from build123d import *

# Parameters (mm, degrees)
SKETCH1_R             = 8
BOSS_EXTRUDE1_DEPTH   = 7
SKETCH2_R             = 6
BOSS_EXTRUDE2_DEPTH   = 7
SKETCH3_R             = 8
BOSS_EXTRUDE3_DEPTH   = 2
CHAMFER1_SIZE         = 0.2
SKETCH4_R             = 2.5
CUT_EXTRUDE1_DEPTH    = 20
BODY_MOVE_COPY1_ANGLE = 180
CUT_EXTRUDE2_DEPTH    = 3


with BuildPart() as part:
    # Sketch1 → Boss-Extrude1 (new body)
    with BuildSketch(Plane(origin=(0, 0, 0), x_dir=(1, 0, 0), z_dir=(0, 1, 0))):
        with Locations(Location((0, 0, 0), (0, 0, 270))):
            Circle(SKETCH1_R)
    extrude(amount=BOSS_EXTRUDE1_DEPTH)

    # Sketch2 → Boss-Extrude2 (add)
    with BuildSketch(Plane(origin=(0, 7, 0), x_dir=(1, 0, 0), z_dir=(0, 1, 0))):
        with Locations(Location((0, 0, 0), (0, 0, 270))):
            Circle(SKETCH2_R)
    extrude(amount=BOSS_EXTRUDE2_DEPTH)

    # Sketch3 → Boss-Extrude3 (add)
    with BuildSketch(Plane(origin=(0, 14, 0), x_dir=(1, 0, 0), z_dir=(0, 1, 0))):
        with Locations(Location((0, 0, 0), (0, 0, 270))):
            Circle(SKETCH3_R)
    extrude(amount=BOSS_EXTRUDE3_DEPTH)

    # Chamfer1
    chamfer1_edges = [part.edges().sort_by_distance(p)[0] for p in [
        (0, 0, -8),
        (0, 7, -8),
        (0, 14, -8),
        (0, 16, -8),
    ]]
    chamfer(chamfer1_edges, length=CHAMFER1_SIZE)

    # Sketch4 → Cut-Extrude1 (cut)
    with BuildSketch(Plane(origin=(0, 16, 0), x_dir=(1, 0, 0), z_dir=(0, 1, 0))):
        with Locations(Location((0, 0, 0), (0, 0, 270))):
            Circle(SKETCH4_R)
    extrude(amount=-CUT_EXTRUDE1_DEPTH, mode=Mode.SUBTRACT)


with BuildPart() as part_1:
    # Body-Move/Copy1: moved
    add(part.part.moved(Location((0, 0, 0))).rotate(Axis((0, 8, 0), (1, 0, 0)), BODY_MOVE_COPY1_ANGLE))

    # Sketch5 → Cut-Extrude2 (cut)
    with BuildSketch(Plane.XZ):
        with BuildLine():
            Line((-4.692804326, 6.230376197), (-7.8, 0))
            ThreePointArc((-7.8, 0), (-9.361590262, 4.668785935), (-4.692804326, 6.230376197))
        make_face()
    extrude(amount=-CUT_EXTRUDE2_DEPTH, mode=Mode.SUBTRACT)


solid = part_1.part
CAD build for the part. Positions are in the model's coordinates, mm. A direction names the side the tool comes from. Round coordinates to 2 decimals unless told otherwise and drop trailing zeros. Write each loop counter-clockwise with the first axis right and the second up, starting at its lowest first coordinate (ties: lowest second). Pieces come first, ordered by that corner, then holes. Notation, with made-up numbers: M -33,-11 L 22,-11 A25 ccw 22,15 Z; hole C 73.5,3 d10. An arc over 180 degrees is marked long. Use a Markdown table: item, result. Add a question column.
1. Pull direction Z, two halves, no side cores. Call faces 3 (the face through (7.02, 1.01, -3.84)), 4 (the face through (-2.44, 7.89, 0.54)), 5 (the face through (-5, 9, -4)): released by +Z, released by -Z, zero draft, split by the parting line, or undercut.
2. Slice it at B-B on y = 2.75. Give the cut face in (x, z).
3. 3-axis set-ups, long thin cutter, end or side, ignore diameter. For faces 1 (the face through (1.802, 5.549, -5.723)), 2 (the face through (2, 0, 2)): which of +Z, -Z, +X, -X, +Y, -Y reach the whole face in a straight line?
4. Drill centre lines: probe 1 along Y at (x, z) = (-0.25, 6.75); probe 2 along X at (y, z) = (5.5, 0); probe 3 along Z at (x, y) = (1.75, 14.25). Where is each one in solid material? Low to high.
5. Slice it at C-C on y = 9.75. Give the cut face in (x, z).
6. Flat gauge pins, fed straight in: P1, Ø3, axis at y = 6, z = 1.5, coming from the -X side; P2, Ø8, axis at y = 13, z = 0.5, coming from the +X side; P3, Ø4, axis at y = 9, z = 6, coming from the +X side; P4, Ø1.5, axis at x = 4, y = 5, coming from the -Z side. Where does each tip first touch, or does it go through?
7. Slice it at A-A on x = 0. Give the cut face in (y, z).
Reply:
| question | item | result |
|---|---|---|
| 1 | face 3 | split by the parting line |
| 1 | face 4 | undercut |
| 1 | face 5 | zero draft |
| 2 | outline | C 0,0 d12; hole C 0,0 d5 |
| 3 | face 1 | none |
| 3 | face 2 | +Z, -Z, +X, -X, -Y |
| 4 | probe 1 | y = 0 to 2, 9 to 16 |
| 4 | probe 2 | x = -6 to -2.5, 2.5 to 6 |
| 4 | probe 3 | z = -7.81 to -1.79, 1.79 to 7.81 |
| 5 | outline | C 0,0 d16; hole C 0,0 d5 |
| 6 | P1 | stops at x = -6 |
| 6 | P2 | stops at x = 8 |
| 6 | P3 | stops at x = 6.92 |
| 6 | P4 | stops at z = -5.04 |
| 7 | outline | M 0,-7.8 L 0.2,-8 L 1.8,-8 L 2,-7.8 L 2,-6 L 9,-6 L 9,-7.8 L 9.2,-8 L 15.8,-8 L 16,-7.8 L 16,-2.5 L 0,-2.5 Z; M 0,2.5 L 16,2.5 L 16,7.8 L 15.8,8 L 9.2,8 L 9,7.8 L 9,6 L 2,6 L 2,7.8 L 1.8,8 L 0.2,8 L 0,7.8 Z |
